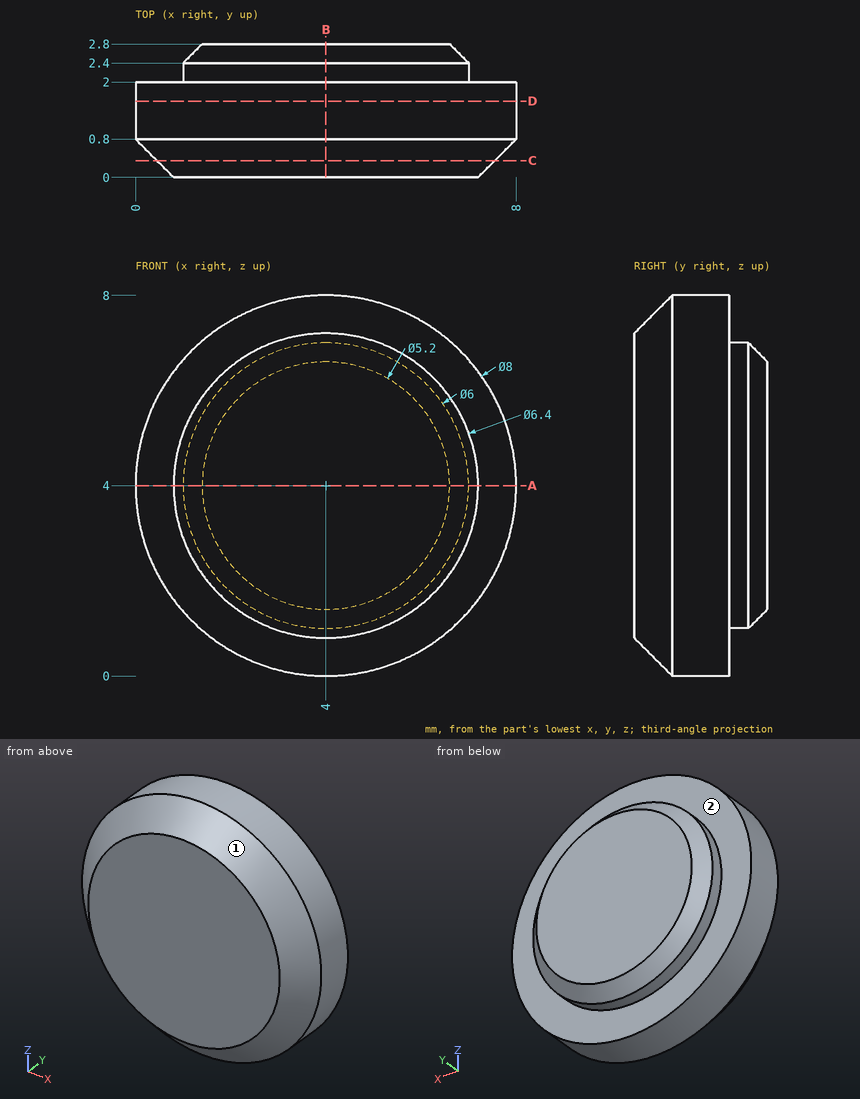
Here's the drawing with two shaded views (mm, measured from the low corner). I have some questions. A direction names the side the tool comes from. Round coordinates to 2 decimals unless told otherwise and drop trailing zeros. Order: outer loops, then holes, each group sorted by start corner. A loop starts at its lowest first (then second) coordinate and runs counter-clockwise, first axis right, second up. Notation, with made-up numbers: (-30, 37) -> (0, 37) arc R19 ccw to (0, 49) -> close; hole circle Ø4 at (-19.75, 2.5). An arc over 180 degrees is marked (long way). Write each question's results on one line, items separated by ' | '. Start each with the question number.
Item 1: If we section it at A-A, the plane z = 4: Write out the boundary of the cut face in (x, y).
Item 2: Please list where these lines run through material, in increasing order: L1, parallel to Y at x = 3, z = 0.75; L2, parallel to Y at x = 6, z = 5.75; L3, parallel to Z at x = 2.25, y = 1.15.
Item 3: If we section it at D-D, the plane y = 1.6: Write out the boundary of the cut face in (x, z), then the cut area to 3 significant figures.
Item 4: Will this pin go through, and if not, where does the flat tip stop? pin 1 (1.5 mm diameter, centred on y = 0.5, z = 7, fed in from -X).
Item 5: If we section it at C-C, the plane y = 0.35: Write out the boundary of the cut face in (x, z), then the cut area to 3 significant figures.
Item 6: Which directions (+Z, -Z, +X, -X, +Y, -Y) give clear straight access to the entire face, cutting with the end or side of a thin tool? Please do the marked faces 1 and 2.
Item 7: If we section it at B-B, the plane x = 4: Write out the boundary of the cut face in (y, z).
Results:
1) outline: (0, 0.8) -> (0.8, 0) -> (7.2, 0) -> (8, 0.8) -> (8, 2) -> (7, 2) -> (7, 2.4) -> (6.6, 2.8) -> (1.4, 2.8) -> (1, 2.4) -> (1, 2) -> (0, 2) -> close
2) L1: y = 0.2 to 2 | L2: y = 0 to 2.74 | L3: z = 0.4 to 7.6
3) outline: circle Ø8 at (4, 4) | area: 50.3 mm2
4) pin 1: stops at x = 0.74
5) outline: circle Ø7.1 at (4, 4) | area: 39.6 mm2
6) face 1: -Y | face 2: +Y
7) outline: (0, 0.8) -> (0.8, 0) -> (2, 0) -> (2, 1) -> (2.4, 1) -> (2.8, 1.4) -> (2.8, 6.6) -> (2.4, 7) -> (2, 7) -> (2, 8) -> (0.8, 8) -> (0, 7.2) -> close
